Build history of the part. All positions in model axes, mm. A direction names the side the tool comes from. Give positions to 0.01 mm unless a question says otherwise; leave off trailing zeros. Loops run counter-clockwise (first coordinate to the right, second up) from the corner with the lowest first, then second, coordinate; pieces in that order, holes last. Notation, with made-up numbers: (7.5, 6.25) - (65.5, 6.25) arc R21 ccw to (65.5, 13.25) - close; hole circle Ø3 at (-22.5, 20). An arc over 180 degrees is marked (long way). Return JSON: item names as keys, results as strings. Group by question number.
1) 3-axis set-ups, long thin cutter, end or side, ignore diameter. For faces 1 (the face through (-0.09, 2.96, -34.25)), 2 (the face through (0, 54, 0)), 3 (the face through (-14, 59, 0)): which of +Z, -Z, +X, -X, +Y, -Y reach the whole face in a straight line?
2) Slice it at C-C (x = 0). List the corners of the cut face in (y, z), and give its area (3 significant figures).
3) Mould opens along Y. For faces 4 (the face through (-10, 30, 3)), 5 (the face through (9, 35, 0)), 6 (the face through (-7, 6, -22)), 7 (the face through (-7, 0, -17)) say: released by +Y, released by -Y, zero draft, split by the parting line, or undercut.
4) Slice it at A-A (z = -10). List the corners of the cut face in (x, y), and give its area (3 significant figures).
5) Slice it at D-D (z = -1.5). List the corners of the cut face in (x, y).
6) Drill centre lines: probe 1 along X at (y, z) = (26, -2); probe 2 along Y at (x, z) = (-12, -12.5); probe 3 along Z at (x, y) = (12.25, 41.5). Where is each one in solid material? Low to high. Write a range as from..to.
7) Slice it at B-B (y = 36). List the corners of the cut face in (x, z), and give its area (3 significant figures).
8) Drop flat-ended pins along their axis: pin 1 (9 mm diameter, centred on x = 5.5, y = 38, fed in from -Z); pin 2 (4 mm diameter, centred on x = -6, z = -31.5, fed in from +Y). Give the stop position or say it passes through.
```python
from build123d import *

# Parameters (mm, degrees)
SKETCH1_W           = 30
SKETCH1_H           = 60
BOSS_EXTRUDE1_DEPTH = 3
SKETCH3_W           = 30
SKETCH3_H           = 34
BOSS_EXTRUDE2_DEPTH = 6
FILLET1_R           = 3
CHAMFER1_SIZE       = 2


with BuildPart() as part:
    # Sketch1 → Boss-Extrude1 (new body, symmetric)
    with BuildSketch(Plane.XY):
        with Locations((0, 30)):
            Rectangle(SKETCH1_W, SKETCH1_H)
        with BuildLine():
            Line((9, 45), (9, 25))
            ThreePointArc((9, 25), (0, 16), (-9, 25))
            Line((-9, 25), (-9, 45))
            ThreePointArc((-9, 45), (0, 54), (9, 45))
        make_face(mode=Mode.SUBTRACT)
    extrude(amount=BOSS_EXTRUDE1_DEPTH, both=True)

    # Sketch3 → Boss-Extrude2 (add)
    with BuildSketch(Plane(origin=(0, 0, 0), x_dir=(1, 0, 0), z_dir=(0, 1, 0))):
        with Locations((0, 20)):
            Rectangle(SKETCH3_W, SKETCH3_H)
        with BuildLine():
            Line((4.25, 30), (4.25, 12))
            ThreePointArc((4.25, 12), (0, 7.75), (-4.25, 12))
            Line((-4.25, 12), (-4.25, 30))
            ThreePointArc((-4.25, 30), (0, 34.25), (4.25, 30))
        make_face(mode=Mode.SUBTRACT)
    extrude(amount=BOSS_EXTRUDE2_DEPTH)

    # Fillet1
    fillet1_edges = [part.edges().sort_by_distance(p)[0] for p in [
        (0, 6, -3),
    ]]
    fillet(fillet1_edges, radius=FILLET1_R)

    # Chamfer1
    chamfer1_edges = [part.edges().sort_by_distance(p)[0] for p in [
        (-15, 3, -37),
        (15, 3, -37),
        (-15, 60, 0),
        (15, 60, 0),
    ]]
    chamfer(chamfer1_edges, length=CHAMFER1_SIZE)


solid = part.part
```
Results:
{
 "1": {"face 1": "+Y, -Y", "face 2": "+Z, -Z", "face 3": "+Z, -Z, -X, +Y"},
 "2": {"outline": "(0, -37) - (6, -37) - (6, -34.25) - (0, -34.25) - close; (0, -7.75) - (6, -7.75) - (6, -6) arc R3 cw to (9, -3) - (16, -3) - (16, 3) - (0, 3) - close; (54, -3) - (60, -3) - (60, 3) - (54, 3) - close", "area": "179 mm2"},
 "3": {"face 4": "zero draft", "face 5": "undercut", "face 6": "released by +Y", "face 7": "released by -Y"},
 "4": {"outline": "(-15, 0) - (-3.75, 0) - (-3.75, 6) - (-15, 6) - close; (3.75, 0) - (15, 0) - (15, 6) - (3.75, 6) - close", "area": "135 mm2"},
 "5": {"outline": "(-15, 0) - (15, 0) - (15, 58) - (13, 60) - (-13, 60) - (-15, 58) - close; hole (-9, 25) arc R9 ccw to (9, 25) - (9, 45) arc R9 ccw to (-9, 45) - close"},
 "6": {"probe 1": "-15..-9, 9..15", "probe 2": "0..6", "probe 3": "-3..3"},
 "7": {"outline": "(-15, -3) - (-9, -3) - (-9, 3) - (-15, 3) - close; (9, -3) - (15, -3) - (15, 3) - (9, 3) - close", "area": "72.0 mm2"},
 "8": {"pin 1": "z = -3", "pin 2": "y = 6"}
}
